Geometry: final body of the model. Coordinates: model frame, mm. Coordinates: 2 decimals unless noted, no trailing zeros. Order: outer loops, then holes, each group sorted by start corner. A loop starts at its lowest first (then second) coordinate and runs counter-clockwise, first axis right, second up. Notation, with made-up numbers: M 1,-38 L 60,-38 A23 cw 60,-10 Z; hole C 20.25,-37 d5. An arc over 180 degrees is marked long. Write item = value, one per line. Start each with the question number.
Autodesk Inventor part; units mm, degrees
ref_plane "YZ Plane" through (0, 0, 0) normal (1, 0, 0) x (0, 1, 0)
ref_plane "XZ Plane" through (0, 0, 0) normal (0, 1, 0) x (-1, 0, 0)
ref_plane "XY Plane" through (0, 0, 0) normal (0, 0, 1) x (1, 0, 0)
ref_plane "Work Plane1" through (139.4467, 111.518, -98.9659) normal (0, 0, -1) x (-1, 0, 0)
sketch "Sketch1" plane through (139.4467, 111.518, -98.9659) normal (0, 0, -1) x (-1, 0, 0)
  line L0 (0, 9.125) -> (0, 18.25)
  line L1 (0, -9.125) -> (0, 0)
  line L2 (-3, -18.25) -> (-3, -9.125)
  line L3 (-3, 0) -> (-3, 9.125)
  line L4 (0, 0) -> (-3, 0)
  line L5 (0, -9.125) -> (-3, -9.125)
  line L6 (0, -18.25) -> (-3, -18.25)
  line L7 (0, -27.375) -> (0, -18.25)
  line L8 (0, 9.125) -> (-3, 9.125)
  line L9 (294, 9.125) -> (294, 18.25)
  line L10 (297, 0) -> (297, 9.125)
  line L11 (294, -9.125) -> (294, 0)
  line L12 (297, -18.25) -> (297, -9.125)
  line L13 (294, -27.375) -> (294, -18.25)
  line L14 (297, -18.25) -> (294, -18.25)
  line L15 (297, -9.125) -> (294, -9.125)
  line L16 (297, 0) -> (294, 0)
  line L17 (297, 9.125) -> (294, 9.125)
  line L18 (0, -27.375) -> (14, -27.375)
  line L19 (14, -27.375) -> (14, -24.375)
  line L20 (14, -24.375) -> (28, -24.375)
  line L21 (28, -24.375) -> (28, -27.375)
  line L22 (56, -24.375) -> (56, -27.375)
  line L23 (42, -24.375) -> (56, -24.375)
  line L24 (42, -27.375) -> (42, -24.375)
  line L25 (28, -27.375) -> (42, -27.375)
  line L26 (84, -24.375) -> (84, -27.375)
  line L27 (70, -24.375) -> (84, -24.375)
  line L28 (70, -27.375) -> (70, -24.375)
  line L29 (56, -27.375) -> (70, -27.375)
  line L30 (112, -24.375) -> (112, -27.375)
  line L31 (98, -24.375) -> (112, -24.375)
  line L32 (98, -27.375) -> (98, -24.375)
  line L33 (84, -27.375) -> (98, -27.375)
  line L34 (140, -24.375) -> (140, -27.375)
  line L35 (126, -24.375) -> (140, -24.375)
  line L36 (126, -27.375) -> (126, -24.375)
  line L37 (112, -27.375) -> (126, -27.375)
  line L38 (168, -24.375) -> (168, -27.375)
  line L39 (154, -24.375) -> (168, -24.375)
  line L40 (154, -27.375) -> (154, -24.375)
  line L41 (140, -27.375) -> (154, -27.375)
  line L42 (196, -24.375) -> (196, -27.375)
  line L43 (182, -24.375) -> (196, -24.375)
  line L44 (182, -27.375) -> (182, -24.375)
  line L45 (168, -27.375) -> (182, -27.375)
  line L46 (224, -24.375) -> (224, -27.375)
  line L47 (210, -24.375) -> (224, -24.375)
  line L48 (210, -27.375) -> (210, -24.375)
  line L49 (196, -27.375) -> (210, -27.375)
  line L50 (252, -24.375) -> (252, -27.375)
  line L51 (238, -24.375) -> (252, -24.375)
  line L52 (238, -27.375) -> (238, -24.375)
  line L53 (224, -27.375) -> (238, -27.375)
  line L54 (280, -24.375) -> (280, -27.375)
  line L55 (266, -24.375) -> (280, -24.375)
  line L56 (266, -27.375) -> (266, -24.375)
  line L57 (252, -27.375) -> (266, -27.375)
  line L58 (280, -27.375) -> (294, -27.375)
  line L59 (0, 18.25) -> (14, 18.25)
  line L60 (14, 18.25) -> (14, 21.25)
  line L61 (14, 21.25) -> (28, 21.25)
  line L62 (28, 21.25) -> (28, 18.25)
  line L63 (56, 21.25) -> (56, 18.25)
  line L64 (42, 21.25) -> (56, 21.25)
  line L65 (42, 18.25) -> (42, 21.25)
  line L66 (28, 18.25) -> (42, 18.25)
  line L67 (84, 21.25) -> (84, 18.25)
  line L68 (70, 21.25) -> (84, 21.25)
  line L69 (70, 18.25) -> (70, 21.25)
  line L70 (56, 18.25) -> (70, 18.25)
  line L71 (112, 21.25) -> (112, 18.25)
  line L72 (98, 21.25) -> (112, 21.25)
  line L73 (98, 18.25) -> (98, 21.25)
  line L74 (84, 18.25) -> (98, 18.25)
  line L75 (140, 21.25) -> (140, 18.25)
  line L76 (126, 21.25) -> (140, 21.25)
  line L77 (126, 18.25) -> (126, 21.25)
  line L78 (112, 18.25) -> (126, 18.25)
  line L79 (168, 21.25) -> (168, 18.25)
  line L80 (154, 21.25) -> (168, 21.25)
  line L81 (154, 18.25) -> (154, 21.25)
  line L82 (140, 18.25) -> (154, 18.25)
  line L83 (196, 21.25) -> (196, 18.25)
  line L84 (182, 21.25) -> (196, 21.25)
  line L85 (182, 18.25) -> (182, 21.25)
  line L86 (168, 18.25) -> (182, 18.25)
  line L87 (224, 21.25) -> (224, 18.25)
  line L88 (210, 21.25) -> (224, 21.25)
  line L89 (210, 18.25) -> (210, 21.25)
  line L90 (196, 18.25) -> (210, 18.25)
  line L91 (252, 21.25) -> (252, 18.25)
  line L92 (238, 21.25) -> (252, 21.25)
  line L93 (238, 18.25) -> (238, 21.25)
  line L94 (224, 18.25) -> (238, 18.25)
  line L95 (280, 21.25) -> (280, 18.25)
  line L96 (266, 21.25) -> (280, 21.25)
  line L97 (266, 18.25) -> (266, 21.25)
  line L98 (252, 18.25) -> (266, 18.25)
  line L99 (280, 18.25) -> (294, 18.25)
  point P0 (139.4467, -111.518)
  point P1 (28, -27.375)
  point P2 (56, -27.375)
  point P3 (168, -27.375)
  point P4 (224, -27.375)
  point P5 (252, 18.25)
  point P6 (224, 18.25)
  point P7 (196, 18.25)
  point P8 (168, 18.25)
  point P9 (140, 18.25)
  point P10 (112, 18.25)
  point P11 (84, 18.25)
  point P12 (56, 18.25)
  point P13 (28, 18.25)
  point P14 (0, 18.25)
  dimension "d0" = 3
  dimension "d1" = 14
  dimension "d4" = 28
  dimension "d13" = 3
  dimension "d14" = 14
  dimension "d15" = 28
extrude "Extrusion1" add sketch "Sketch1" along normal blind 3
sketch "Sketch2" plane through (139.4467, 111.518, -101.9659) normal (0, 0, -1) x (-1, 0, 0)
  line L0 (107, 6.9375) -> (187, 6.9375)
  line L1 (187, 6.9375) -> (187, -13.0625)
  line L2 (187, -13.0625) -> (107, -13.0625)
  line L3 (107, -13.0625) -> (107, 6.9375)
  line L4 (187, -3.0625) -> (294, -3.0625) construction
  line L5 (294, -9.125) -> (294, 0)
  line L6 (107, -3.0625) -> (0, -3.0625) construction
  line L7 (0, 0) -> (0, -9.125)
  line L8 (147, -13.0625) -> (147, -24.375) construction
  line L9 (154, -24.375) -> (168, -24.375)
  line L10 (147, 6.9375) -> (147, 18.25) construction
  line L11 (154, 18.25) -> (140, 18.25)
  point P0 (139.4467, -111.518)
  dimension "d19" = 80
  dimension "d20" = 20
extrude "Extrusion2" cut sketch "Sketch2" against normal blind 3
properties part number "BackWall"
Item 1: Draft query along Z for faces 1 (the flat face through (-5, 98, -101.966)), 2 (the flat face through (-5, 98, -98.966)). Return one class per face: pulls with the +Z half, pulls with the -Z half, needs draft (parallel to the pull), parting line crosses it, or undercut.
Item 2: Section query A-A on x = -7. Output: boundary loops of the cut face in (y, z), and give its area (3 significant figures).
Item 3: Section query B-B on y = 116. Output: boundary loops of the cut face in (x, z), and give its area (3 significant figures).
Item 4: Section query C-C on x = -120.5. Output: boundary loops of the cut face in (y, z).
Item 5: Material intervals for probe 1 along Y at (x, z) = (-23.5, -100.1); probe 2 along X at (y, z) = (103, -101.35); probe 3 along Y at (x, z) = (-8, -100.05), sorted ascending. Write a range as [from, to].
Item 6: First-contact query: pin 1 (1.5 mm diameter, centred on y = 86, z = -100, fed in from -X); pin 2 (1.5 mm diameter, centred on x = 23, z = -101, fed in from +Y); pin 3 (1.5 mm diameter, centred on x = 140.5, z = -100.5, fed in from +Y). Flat tips, straight axial feed; report the tip coordinate or a pass-through.
Ans:
q1.face_1 = pulls with the -Z half
q1.face_2 = pulls with the +Z half
q2.outline = M 84.14,-101.97 L 98.46,-101.97 L 98.46,-98.97 L 84.14,-98.97 Z; M 118.46,-101.97 L 129.77,-101.97 L 129.77,-98.97 L 118.46,-98.97 Z
q2.area = 76.9 mm^2
q3.outline = M -157.55,-101.97 L -47.55,-101.97 L -47.55,-98.97 L -157.55,-98.97 Z; M 32.45,-101.97 L 142.45,-101.97 L 142.45,-98.97 L 32.45,-98.97 Z
q3.area = 660 mm^2
q4.outline = M 84.14,-101.97 L 129.77,-101.97 L 129.77,-98.97 L 84.14,-98.97 Z
q5.probe_1 = [87.14, 98.46], [118.46, 132.77]
q5.probe_2 = [-154.55, -47.55], [32.45, 139.45]
q5.probe_3 = [84.14, 98.46], [118.46, 129.77]
q6.pin_1 = -154.55
q6.pin_2 = 129.77
q6.pin_3 = 120.64
